from build123d import *

# Parameters (mm, degrees)
SKETCH1_W            = 45
SKETCH1_H            = 60
BOSS_EXTRUDE1_DEPTH  = 11
SKETCH6_R            = 2.75
CUT_EXTRUDE2_DEPTH   = 8.5
CUT_EXTRUDE3_DEPTH   = 40.080046059
SKETCH11_W           = 45
SKETCH11_H           = 11
BOSS_EXTRUDE2_DEPTH  = 6
M4_CLEARANCE_HOLE2_D = 4.8
FILLET1_R            = 10


with BuildPart() as part:
    # Sketch1 → Boss-Extrude1 (new body)
    with BuildSketch(Plane.XY):
        Rectangle(SKETCH1_W, SKETCH1_H)
    boss_extrude1 = extrude(amount=-BOSS_EXTRUDE1_DEPTH)

    # Sketch6 → Cut-Extrude2 (cut)
    with BuildSketch(Plane.XY):
        with Locations((-16, 16)):
            Circle(SKETCH6_R)
        with Locations((16, 16)):
            Circle(SKETCH6_R)
        with Locations((16, -16)):
            Circle(SKETCH6_R)
        with Locations((-16, -16)):
            Circle(SKETCH6_R)
    cut_extrude2 = extrude(amount=-CUT_EXTRUDE2_DEPTH, mode=Mode.SUBTRACT)

    # Sketch7 → Cut-Extrude3 (cut, through all)
    with BuildSketch(Plane.XY):
        with BuildLine():
            ThreePointArc((19, 0), (0, 19), (-19, 0))
            ThreePointArc((-19, 0), (0, -19), (19, 0))
        make_face()
    cut_extrude3 = extrude(amount=-CUT_EXTRUDE3_DEPTH, mode=Mode.SUBTRACT)

    # Sketch11 → Boss-Extrude2 (add)
    with BuildSketch(Plane.XZ.offset(30)):
        with Locations((0, -5.5)):
            Rectangle(SKETCH11_W, SKETCH11_H)
    extrude(amount=BOSS_EXTRUDE2_DEPTH)

    # Mirror1: Boss-Extrude1, Cut-Extrude2, Cut-Extrude3 across plane
    add(boss_extrude1.mirror(Plane(origin=(0, -33, 0), x_dir=(0, 0, 1), z_dir=(0, -1, 0))))
    add(cut_extrude2.mirror(Plane(origin=(0, -33, 0), x_dir=(0, 0, 1), z_dir=(0, -1, 0))), mode=Mode.SUBTRACT)
    add(cut_extrude3.mirror(Plane(origin=(0, -33, 0), x_dir=(0, 0, 1), z_dir=(0, -1, 0))), mode=Mode.SUBTRACT)

    # M4 Clearance Hole2 (through all)
    with Locations(Plane.XY):
        with Locations((0, -91), (0, -33), (0, 25)):
            Hole(M4_CLEARANCE_HOLE2_D / 2)

    # Fillet1
    fillet1_edges = [part.edges().sort_by_distance(p)[0] for p in [
        (22.5, -96, -5.5),
        (-22.5, -96, -5.5),
        (-22.5, 30, -5.5),
        (22.5, 30, -5.5),
    ]]
    fillet(fillet1_edges, radius=FILLET1_R)


solid = part.part
Could you check a few things on this model? Use its own coordinates, in mm. A direction names the side the tool comes from. Coordinates: 2 decimals unless noted, no trailing zeros. Order: outer loops, then holes, each group sorted by start corner. A loop starts at its lowest first (then second) coordinate and runs counter-clockwise, first axis right, second up. Notation, with made-up numbers: (-15.5, 55) -> (-5.5, 55) arc R20 cw to (-5.5, 81) -> close; hole circle Ø3 at (77.25, 50.5). An arc over 180 degrees is marked (long way). One line per item, written item: value. Start each with the question number.
1) Imagine slicing it at A-A on y = -33. List the corners of the cut face in (x, z) for me.
2) I'm going to push a flat-ended pin straight in: pin 1 (3 mm diameter, centred on x = 0, y = 25, fed in from +Z). Where does the tip first touch, or does it pass through?
3) If I drill on L1, parallel to Y at x = 0, z = -5.25; L2, parallel to X at y = -82, z = -2.5; L3, parallel to Y at x = 4, z = -8, over which ranges is the centre line in solid material (lowest first)? Write a range as [from, to].
4) Imagine slicing it at B-B on x = -16. List the corners of the cut face in (y, z) for me.
5) Imagine slicing it at C-C on z = -4.5. Count the separate pieces of the cut face and the enclosed holes in it, plus the area to 3 significant figures.
6) Imagine slicing it at D-D on x = 0. List the corners of the cut face in (y, z) for me.
7) Which directions (+Z, -Z, +X, -X, +Y, -Y) give clear straight access to the entire face, cutting with the end or side of a thin tool? Please do faces 1 (the cylindrical face through (-19.65, -92.99, -5.58)), 2 (the cylindrical face through (13.253, -15.879, -4.19)).
Answer list:
1. outline: (-22.5, -11) -> (-2.4, -11) -> (-2.4, 0) -> (-22.5, 0) -> close; (2.4, -11) -> (22.5, -11) -> (22.5, 0) -> (2.4, 0) -> close
2. pin 1: passes through
3. L1: y = [-96, -93.4], [-88.6, -85], [-47, -35.4], [-30.6, -19], [19, 22.6], [27.4, 30]
3. L2: x = [-22.5, -18.75], [-13.25, -10.25], [10.25, 13.25], [18.75, 22.5]
3. L3: y = [-96, -84.57], [-47.43, -18.57], [18.57, 30]
4. outline: (-95.37, -11) -> (-76.25, -11) -> (-76.25, 0) -> (-79.25, 0) -> (-79.25, -8.5) -> (-84.75, -8.5) -> (-84.75, 0) -> (-95.37, 0) -> close; (-55.75, -11) -> (-10.25, -11) -> (-10.25, 0) -> (-13.25, 0) -> (-13.25, -8.5) -> (-18.75, -8.5) -> (-18.75, 0) -> (-47.25, 0) -> (-47.25, -8.5) -> (-52.75, -8.5) -> (-52.75, 0) -> (-55.75, 0) -> close; (10.25, -11) -> (29.37, -11) -> (29.37, 0) -> (18.75, 0) -> (18.75, -8.5) -> (13.25, -8.5) -> (13.25, 0) -> (10.25, 0) -> close
5. separate pieces: 1
5. enclosed holes: 13
5. area: 3,070 mm2
6. outline: (-96, -11) -> (-93.4, -11) -> (-93.4, 0) -> (-96, 0) -> close; (-88.6, -11) -> (-85, -11) -> (-85, 0) -> (-88.6, 0) -> close; (-47, -11) -> (-35.4, -11) -> (-35.4, 0) -> (-47, 0) -> close; (-30.6, -11) -> (-19, -11) -> (-19, 0) -> (-30.6, 0) -> close; (19, -11) -> (22.6, -11) -> (22.6, 0) -> (19, 0) -> close; (27.4, -11) -> (30, -11) -> (30, 0) -> (27.4, 0) -> close
7. face 1: +Z, -Z, -X, -Y
7. face 2: +Z
